from build123d import *


with BuildPart() as part:
    # Sketch1 → Revolve1 (revolve)
    with BuildSketch(Plane.XY):
        with BuildLine():
            Line((0, -6), (4.95, -6))
            ThreePointArc((4.95, -6), (5.657106781, -5.707106781), (5.95, -5))
            Line((5.95, -5), (5.95, -2))
            Line((5.95, -2), (9, -2))
            ThreePointArc((9, -2), (8.807077454, -0.932475563), (8.252715788, 0))
            Line((8.252715788, 0), (5, 0))
            ThreePointArc((5, 0), (4.292893219, -0.292893219), (4, -1))
            Line((4, -1), (4, -3))
            Line((4, -3), (0, -3))
            Line((0, -3), (0, -6))
        make_face()
    revolve(axis=Axis((0, 0, 0), (0, -1, 0)))


solid = part.part
Verification items for the finished model (mm, model axes). A direction names the side the tool comes from. Give positions to 0.01 mm unless a question says otherwise; leave off trailing zeros. Write each loop counter-clockwise with the first axis right and the second up, starting at its lowest first coordinate (ties: lowest second). Pieces come first, ordered by that corner, then holes. Notation, with made-up numbers: M 31,-13.75 L 89,-13.75 A25 ccw 89,-1.75 Z; hole C 89,89 d1. An arc over 180 degrees is marked long. Put each result on its own line as item: value. Start each with the question number.
1. Go/stop test with flat-tipped pins: pin 1 Ø3 at (x, y) = (6.5, -5) entering from +Z; pin 2 Ø3 at (y, z) = (-1.5, -4.5) entering from +X; pin 3 Ø2 at (y, z) = (-2.5, -6.5) entering from -X. Record where each tip stops, or that it passes through.
2. Section check B-B (x = 0). Record the cut outline in (y, z), and give its area (3 significant figures).
3. Draft check along X on faces 1 (the face through (-4.385, -3.479, 4.021)), 2 (the face through (-0.867, -2.014, -3.905)), 3 (the face through (-2, -2, -6)). Enter one of: +X half, -X half, draft (parallel to the pull), parting line (faces both ways), or undercut.
4. Section check C-C (y = -2.75). Record the cut outline in (x, z), and give its area (3 significant figures).
5. Set-up check for faces 4 (the face through (4, 0, -4)), 5 (the face through (0, -3, 0)): record each of +Z, -Z, +X, -X, +Y, -Y from which the full face is reachable in a straight line by a thin tool's end or side.
6. Scan lines: line 1 along Z through (x, y) = (0, -2.15); line 2 along Y through (x, z) = (2, -1.75); line 3 along Z through (x, y) = (0, -1.9). Record each from-to range of solid material in increasing order. Write a range as [from, to].
7. Section check A-A (z = 0). Record the cut outline in (x, y), and give its area (3 significant figures).
8. Section check D-D (y = -4.1). Record the cut outline in (x, z), and give its area (3 significant figures).
Answer list:
1. pin 1: z = 3.23
1. pin 2: x = 8.47
1. pin 3: x = -7.02
2. outline: M -6,-4.95 A1 ccw -5,-5.95 L -2,-5.95 L -2,-9 A3.05 ccw 0,-8.25 L 0,-5 A1 ccw -1,-4 L -3,-4 L -3,4 L -1,4 A1 ccw 0,5 L 0,8.25 A3.05 ccw -2,9 L -2,5.95 L -5,5.95 A1 ccw -6,4.95 Z
2. area: 57.8 mm2
3. face 1: parting line
3. face 2: undercut
3. face 3: draft
4. outline: C 0,0 d11.9; hole C 0,0 d8
4. area: 61.0 mm2
5. face 4: +Z, -Z, +X, -X, +Y
5. face 5: +Y
6. line 1: [-5.95, -4], [4, 5.95]
6. line 2: [-6, -3]
6. line 3: [-9, -4], [4, 9]
7. outline: M -9,-2 L -5.95,-2 L -5.95,-5 A1 ccw -4.95,-6 L 4.95,-6 A1 ccw 5.95,-5 L 5.95,-2 L 9,-2 A3.05 ccw 8.25,0 L 5,0 A1 ccw 4,-1 L 4,-3 L -4,-3 L -4,-1 A1 ccw -5,0 L -8.25,0 A3.05 ccw Z
7. area: 57.8 mm2
8. outline: C 0,0 d11.9
8. area: 111 mm2
